Design review of the part built by this model. Coordinates are the model's own, in mm. A direction names the side the tool comes from. Coordinates: 2 decimals unless noted, no trailing zeros. Order: outer loops, then holes, each group sorted by start corner. A loop starts at its lowest first (then second) coordinate and runs counter-clockwise, first axis right, second up. Notation, with made-up numbers: (-26, 27) -> (-11, 27) arc R23 ccw to (-11, 49) -> close; hole circle Ø3 at (-18.5, 21.5). An arc over 180 degrees is marked (long way). Write item = value, one per line.
```python
from build123d import *

# Parameters (mm, degrees)
SKETCH1_R           = 17
SKETCH1_R_2         = 12.5
BOSS_EXTRUDE1_DEPTH = 4
SKETCH2_R           = 1.55
CUT_EXTRUDE1_DEPTH  = 25.372115214
BOSS_EXTRUDE2_START = -2
SKETCH3_R           = 12.5
SKETCH3_R_2         = 10.5
BOSS_EXTRUDE2_DEPTH = 2
CHAMFER1_SIZE       = 0.2
CHAMFER2_SIZE       = 0.4


with BuildPart() as part:
    # Sketch1 → Boss-Extrude1 (new body)
    with BuildSketch(Plane(origin=(0, 0, 0), x_dir=(1, 0, 0), z_dir=(0, 1, 0))):
        with Locations(Location((0, 0, 0), (0, 0, 270))):
            Circle(SKETCH1_R)
        with Locations(Location((0, 0, 0), (0, 0, 270))):
            Circle(SKETCH1_R_2, mode=Mode.SUBTRACT)
    extrude(amount=BOSS_EXTRUDE1_DEPTH)

    # Sketch2 → Cut-Extrude1 (cut, through all)
    with BuildSketch(Plane(origin=(0, 4, 0), x_dir=(1, 0, 0), z_dir=(0, 1, 0))):
        with Locations(Location((-8.485, 12.005347771, 0), (0, 0, 270))):
            Circle(SKETCH2_R)
        with Locations(Location((6.154436151, 13.350899437, 0), (0, 0, 270))):
            Circle(SKETCH2_R)
        with Locations(Location((14.639436151, 1.345551666, 0), (0, 0, 270))):
            Circle(SKETCH2_R)
        with Locations(Location((8.485, -12.005347771, 0), (0, 0, 270))):
            Circle(SKETCH2_R)
        with Locations(Location((-6.154436151, -13.350899437, 0), (0, 0, 270))):
            Circle(SKETCH2_R)
        with Locations(Location((-14.639436151, -1.345551666, 0), (0, 0, 270))):
            Circle(SKETCH2_R)
        Polygon((-8.485, 14.731081936), (6.154436151, 15.846858227), (5.945678869, 18.585838188), (-8.485, 17.485972785), align=None)
        Polygon((8.485, -14.731081936), (8.693757282, -17.470061897), (-5.736921587, -18.5699273), (-6.154436151, -15.846858227), align=None)
    extrude(amount=-CUT_EXTRUDE1_DEPTH, mode=Mode.SUBTRACT)

    # Sketch3 → Boss-Extrude2 (add)
    with BuildSketch(Plane(origin=(0, 4, 0), x_dir=(1, 0, 0), z_dir=(0, 1, 0)).offset(BOSS_EXTRUDE2_START)):
        with Locations(Location((0, 0, 0), (0, 0, 270))):
            Circle(SKETCH3_R)
        with Locations(Location((0, 0, 0), (0, 0, 270))):
            Circle(SKETCH3_R_2, mode=Mode.SUBTRACT)
    extrude(amount=BOSS_EXTRUDE2_DEPTH)

    # Chamfer1
    chamfer1_edges = [part.edges().sort_by_distance(p)[0] for p in [
        (0, 0, -12.5),
        (0, 2, -12.5),
        (0, 2, -10.5),
    ]]
    chamfer(chamfer1_edges, length=CHAMFER1_SIZE)

    # Chamfer2
    chamfer2_edges = [part.edges().sort_by_distance(p)[0] for p in [
        (-16.950837114, 0, 1.291944715),
        (16.950837114, 0, -1.291944715),
        (-1.165281924, 0, -15.288970081),
        (1.165281924, 0, 15.288970081),
    ]]
    chamfer(chamfer2_edges, length=CHAMFER2_SIZE)


solid = part.part
```
(1) For L1, parallel to Z at x = -8.5, y = 3.35; L2, parallel to Z at x = 6.5, y = 3.35; L3, parallel to X at y = 0.35, z = -11, list the stretches that pass through material, from the lowest coordinate up.
Report:
L1 = -14.72 to -13.56, -10.46 to -6.16, 6.16 to 14.72
L2 = -15.71 to -14.86, -11.84 to -8.25, 8.25 to 14.88
L3 = -12.9 to -9.66, -7.31 to -5.94, 5.94 to 12.9
(2) We need section B-B (y = 2.8). Write out the cut boundary in (x, z) (3 decimals), and give its area (3 significant figures).
Report:
outline = (-8.485, -14.731) -> (6.154, -15.847) arc R17 ccw to (8.485, 14.731) -> (-6.154, 15.847) arc R17 ccw to start; hole circle Ø3.1 at (-14.639, 1.346); hole circle Ø21 at (0, 0); hole circle Ø3.1 at (-8.485, -12.005); hole circle Ø3.1 at (-6.154, 13.351); hole circle Ø3.1 at (6.154, -13.351); hole circle Ø3.1 at (8.485, 12.005); hole circle Ø3.1 at (14.639, -1.346)
area = 483 mm²
(3) We need section C-C (y = 0.8). Write out the cut boundary in (x, z) (3 decimals), and give its area (3 significant figures).
Report:
outline = (-8.485, -14.731) -> (6.154, -15.847) arc R17 ccw to (8.485, 14.731) -> (-6.154, 15.847) arc R17 ccw to start; hole circle Ø3.1 at (-14.639, 1.346); hole circle Ø25 at (0, 0); hole circle Ø3.1 at (-8.485, -12.005); hole circle Ø3.1 at (-6.154, 13.351); hole circle Ø3.1 at (6.154, -13.351); hole circle Ø3.1 at (8.485, 12.005); hole circle Ø3.1 at (14.639, -1.346)
area = 339 mm²
(4) For faces 5 (the cylindrical face through (13.126, 2.028, -1.682)), 6 (the cylindrical face through (3.755, 0.989, 11.923)), list the 3-axis set-ups (+Z, -Z, +X, -X, +Y, -Y) from which the entire face can be reached by the end or side of a thin tool; tool diameter is ignored.
Report:
face_5 = +Y, -Y
face_6 = -Y
(5) We need section A-A (x = 0). Write out the cut boundary in (y, z), and give its area (3 significant figures).
Report:
outline = (0, -14.98) -> (0.4, -15.38) -> (4, -15.38) -> (4, -10.5) -> (2.2, -10.5) -> (2, -10.7) -> (2, -12.3) -> (1.8, -12.5) -> (0.2, -12.5) -> (0, -12.7) -> close; (0, 12.7) -> (0.2, 12.5) -> (1.8, 12.5) -> (2, 12.3) -> (2, 10.7) -> (2.2, 10.5) -> (4, 10.5) -> (4, 15.38) -> (0.4, 15.38) -> (0, 14.98) -> close
area = 30.8 mm²
(6) The part is to be moulded in two halves that separate along Z. For faces 1 (the flat face through (1, 0.2, 15.1)), 2 (the flat face through (-11, 2, -1)), 3 (the cylindrical face through (-9.079, 2.028, -10.574)), 4 (the flat face through (-1.27, 2.23, -15.28)), say which applies: released by +Z, released by -Z, zero draft, split by the parting line, or undercut.
Report:
face_1 = released by +Z
face_2 = undercut
face_3 = undercut
face_4 = released by -Z
(7) Insertion check: pin 1 (1 mm diameter, centred on x = -4.5, z = -10, fed in from -Y); pin 2 (4 mm diameter, centred on x = 14.64, z = -1.35, fed in from -Y). Each pin has a flat end and moves straight along its axis. Give the tip position at first contact, or say it passes through.
Report:
pin_1 = 2
pin_2 = 0
